from build123d import *

# Parameters (mm, degrees)
SKETCH1_R           = 35
SKETCH1_R_2         = 7.5
BOSS_EXTRUDE2_DEPTH = 2.5
BOSS_EXTRUDE3_START = 5
SKETCH1_10_R        = 37.5
SKETCH1_10_R_2      = 35
SKETCH1_10_R_3      = 7.5
BOSS_EXTRUDE3_DEPTH = 2.5
BOSS_EXTRUDE4_START = -2.5
SKETCH1_11_R        = 37.5
SKETCH1_11_R_2      = 35
BOSS_EXTRUDE4_DEPTH = 2.5
BOSS_EXTRUDE6_START = -5
SKETCH1_15_R        = 35
SKETCH1_15_R_2      = 7.5
BOSS_EXTRUDE6_DEPTH = 2.5
SKETCH1_16_R        = 7.5
SKETCH1_16_R_2      = 5
BOSS_EXTRUDE7_DEPTH = 5


with BuildPart() as part:
    # Sketch1 → Boss-Extrude2 (new, symmetric)
    with BuildSketch(Plane(origin=(0, 0, 0), x_dir=(1, 0, 0), z_dir=(0, 1, 0))):
        with Locations(Location((0, 0, 0), (0, 0, 270))):
            Circle(SKETCH1_R)
        with Locations(Location((0, 0, 0), (0, 0, 270))):
            Circle(SKETCH1_R_2, mode=Mode.SUBTRACT)
    extrude(amount=BOSS_EXTRUDE2_DEPTH, both=True)

    # Sketch1<10> → Boss-Extrude3 (add)
    # profile 1 of 2: a face of its own
    with BuildSketch(Plane(origin=(0, 0, 0), x_dir=(1, 0, 0), z_dir=(0, 1, 0)).offset(BOSS_EXTRUDE3_START)):
        with Locations(Location((0, 0, 0), (0, 0, 270))):
            Circle(SKETCH1_10_R)
        with Locations(Location((0, 0, 0), (0, 0, 270))):
            Circle(SKETCH1_10_R_2, mode=Mode.SUBTRACT)
    # profile 2 of 2: a face of its own
    with BuildSketch(Plane(origin=(0, 0, 0), x_dir=(1, 0, 0), z_dir=(0, 1, 0)).offset(BOSS_EXTRUDE3_START)):
        with Locations(Location((0, 0, 0), (0, 0, 270))):
            Circle(SKETCH1_10_R_2)
        with Locations(Location((0, 0, 0), (0, 0, 270))):
            Circle(SKETCH1_10_R_3, mode=Mode.SUBTRACT)
    extrude(amount=-BOSS_EXTRUDE3_DEPTH)



with BuildPart() as body_2:
    # Sketch1<11> → Boss-Extrude4 (new body)
    with BuildSketch(Plane(origin=(0, 0, 0), x_dir=(1, 0, 0), z_dir=(0, 1, 0)).offset(BOSS_EXTRUDE4_START)):
        with Locations(Location((0, 0, 0), (0, 0, 270))):
            Circle(SKETCH1_11_R)
        with Locations(Location((0, 0, 0), (0, 0, 270))):
            Circle(SKETCH1_11_R_2, mode=Mode.SUBTRACT)
    extrude(amount=-BOSS_EXTRUDE4_DEPTH)


with BuildPart() as part_1:
    add(part.part)

    add(body_2.part)  # Boss-Extrude6 merges body 2
    # Sketch1<15> → Boss-Extrude6 (add)
    with BuildSketch(Plane(origin=(0, 0, 0), x_dir=(1, 0, 0), z_dir=(0, 1, 0)).offset(BOSS_EXTRUDE6_START)):
        with Locations(Location((0, 0, 0), (0, 0, 270))):
            Circle(SKETCH1_15_R)
        with Locations(Location((0, 0, 0), (0, 0, 270))):
            Circle(SKETCH1_15_R_2, mode=Mode.SUBTRACT)
    extrude(amount=BOSS_EXTRUDE6_DEPTH)

    # Sketch1<16> → Boss-Extrude7 (add, symmetric)
    with BuildSketch(Plane(origin=(0, 0, 0), x_dir=(1, 0, 0), z_dir=(0, 1, 0))):
        Circle(SKETCH1_16_R)
        with Locations(Location((0, 0, 0), (0, 0, 270))):
            Circle(SKETCH1_16_R_2, mode=Mode.SUBTRACT)
    extrude(amount=BOSS_EXTRUDE7_DEPTH, both=True)


solid = part_1.part
The listing builds one solid part. Answer for the finished solid, in the listing's coordinates (mm). A direction names the side the tool comes from. Give positions to 0.01 mm unless a question says otherwise; leave off trailing zeros. Write each loop counter-clockwise with the first axis right and the second up, starting at its lowest first coordinate (ties: lowest second). Pieces come first, ordered by that corner, then holes.
1) Section C-C (y = 4) is taken. Write down the section's boundary in (x, z).
2) A tool of negligible diameter and unlimited length cuts with its end or side. For faces 4 (the face through (17, -2.5, -31)), 5 (the face through (-1, -5, 8)), from which of +Z, -Z, +X, -X, +Y, -Y can it reach the whole face along a straight path? Write none if from no direction.
3) Find the intervals of material crossed by L1, parallel to X at y = 1, z = 0; L2, parallel to X at y = -2.75, z = 0; L3, parallel to Y at x = -27.5, z = 24.5, in increasing order.
4) For a pull along X with two mould halves and no side action, classify faces 1 (the face through (-22.818, -3.732, -29.759)), 2 (the face through (-1, 5, 8)), 3 (the face through (-4.88, -0.07, -1.08)) as pulls with the +X half, pulls with the -X half, needs draft (parallel to the pull), parting line crosses it, or undercut.
5) Section D-D (x = -8) is taken. Write down the section's boundary in (y, z).
6) Section B-B (z = 0) is taken. Write down the section's boundary in (x, y).
7) Given P1, Ø1, axis at x = -14.5, y = -4, coming from the +Z side; P2, Ø2, axis at x = -10.5, y = -0.5, coming from the -Z side; P3, Ø6, axis at y = 1, z = -27.5, coming from the -X side, each flat-ended and moving along its own axis, determine where each tip first touches the part or whether it passes through.
8) Section A-A (x = 0) is taken. Write down the section's boundary in (y, z).
Response:
1. outline: circle Ø75 at (0, 0); hole circle Ø10 at (0, 0)
2. face 4: none
2. face 5: +Z, -Z, +X, -X, -Y
3. L1: x = -35 to -5, 5 to 35
3. L2: x = -37.5 to -5, 5 to 37.5
3. L3: y = -5 to -2.5, 2.5 to 5
4. face 1: parting line crosses it
4. face 2: needs draft
4. face 3: undercut
5. outline: (-5, -36.64) - (-2.5, -36.64) - (-2.5, -34.07) - (2.5, -34.07) - (2.5, -36.64) - (5, -36.64) - (5, 36.64) - (2.5, 36.64) - (2.5, 34.07) - (-2.5, 34.07) - (-2.5, 36.64) - (-5, 36.64) - close
6. outline: (-37.5, -5) - (-5, -5) - (-5, 5) - (-37.5, 5) - (-37.5, 2.5) - (-35, 2.5) - (-35, -2.5) - (-37.5, -2.5) - close; (5, -5) - (37.5, -5) - (37.5, -2.5) - (35, -2.5) - (35, 2.5) - (37.5, 2.5) - (37.5, 5) - (5, 5) - close
7. P1: stops at z = 34.79
7. P2: stops at z = -33.69
7. P3: stops at x = -28.04
8. outline: (-5, -37.5) - (-2.5, -37.5) - (-2.5, -35) - (2.5, -35) - (2.5, -37.5) - (5, -37.5) - (5, -5) - (-5, -5) - close; (-5, 5) - (5, 5) - (5, 37.5) - (2.5, 37.5) - (2.5, 35) - (-2.5, 35) - (-2.5, 37.5) - (-5, 37.5) - close
